Read the model definition and answer for the solid it produces. Units are mm, in the model's axes. Face numbers are marked on the shaded views. A direction names the side the tool comes from. Give positions to 0.01 mm unless a question says otherwise; leave off trailing zeros. Order: outer loops, then holes, each group sorted by start corner. A loop starts at its lowest first (then second) coordinate and runs counter-clockwise, first axis right, second up. Notation, with made-up numbers: (3, -11) - (16, -11) arc R18 cw to (16, 11) - close; hole circle Ø2 at (-3.75, 72). An arc over 180 degrees is marked (long way). Return JSON: item names as keys, results as strings.
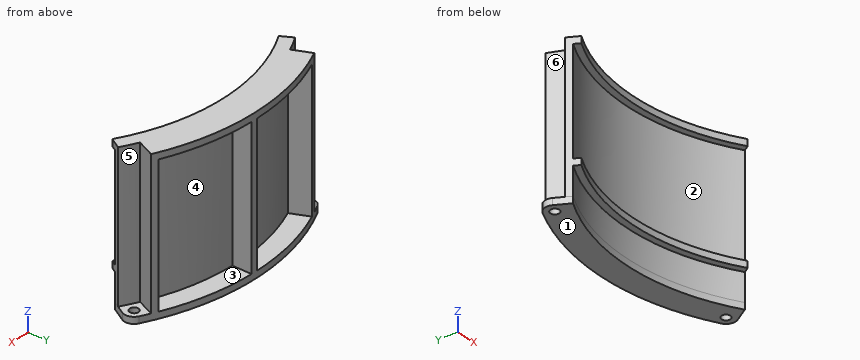
```python
from build123d import *

# Parameters (mm, degrees)
F1_DEPTH = 70.64375
F2_W     = 3.175
F2_H     = 50.8
F2_H_2   = 13.49375
F5_DEPTH = 70.64375
F6_R     = 2.15265
F7_DEPTH = 3.175
F9_DEPTH = 3.175


with BuildPart() as f1:
    # F0 (on Top) → F1 (new body)
    with BuildSketch(Plane.XY):
        with BuildLine():
            ThreePointArc((-49.2125, 85.2385503675), (0, 98.425), (49.2125, 85.2385503675))
            Line((49.2125, 85.2385503675), (57.15, 98.9867036526))
            ThreePointArc((57.15, 98.9867036526), (0, 114.3), (-57.15, 98.9867036526))
            Line((-57.15, 98.9867036526), (-49.2125, 85.2385503675))
        make_face()
    extrude(amount=F1_DEPTH)

    # F2 (on face) → F3 (revolve, cut)
    with BuildSketch(Plane(origin=(0, 0, 0), x_dir=(0.5, -0.8660254038, 0), z_dir=(-0.8660254038, -0.5, 0))):
        with Locations((-100.0125, 42.06875)):
            Rectangle(F2_W, F2_H)
        with Locations((-100.0125, 6.746875)):
            Rectangle(F2_W, F2_H_2)
    revolve(axis=Axis((0, 0, 0), (0, 0, -1)), mode=Mode.SUBTRACT)

    # F4 (on face) → F5 (cut, through all)
    with BuildSketch(Plane.XY.offset(70.64375)):
        with BuildLine():
            ThreePointArc((-48.2700740152, 103.6073836875), (-52.7606451092, 101.3943012583), (-57.15, 98.9867036526))
            Line((-57.15, 98.9867036526), (-52.3875, 90.7378116815))
            ThreePointArc((-52.3875, 90.7378116815), (-48.4225984878, 92.9142216277), (-44.3674611423, 94.9174853059))
            Line((-44.3674611423, 94.9174853059), (-48.2700740152, 103.6073836875))
        make_face()
        with BuildLine():
            Line((-45.3737460178, 104.9081177617), (-41.4711331449, 96.2182193801))
            ThreePointArc((-41.4711331449, 96.2182193801), (-21.9491383614, 102.4501632512), (-1.5875, 104.7629727945))
            Line((-1.5875, 104.7629727945), (-1.5875, 114.2889751627))
            ThreePointArc((-1.5875, 114.2889751627), (-23.944514576, 111.7638144558), (-45.3737460178, 104.9081177617))
        make_face()
        with BuildLine():
            Line((1.5875, 114.2889751627), (1.5875, 104.7629727945))
            ThreePointArc((1.5875, 104.7629727945), (21.9491383614, 102.4501632512), (41.4711331449, 96.2182193801))
            Line((41.4711331449, 96.2182193801), (45.3737460178, 104.9081177617))
            ThreePointArc((45.3737460178, 104.9081177617), (23.944514576, 111.7638144558), (1.5875, 114.2889751627))
        make_face()
        with BuildLine():
            ThreePointArc((44.3674611423, 94.9174853059), (48.4225984878, 92.9142216277), (52.3875, 90.7378116815))
            Line((52.3875, 90.7378116815), (57.15, 98.9867036526))
            ThreePointArc((57.15, 98.9867036526), (52.7606451092, 101.3943012583), (48.2700740152, 103.6073836875))
            Line((48.2700740152, 103.6073836875), (44.3674611423, 94.9174853059))
        make_face()
    extrude(amount=-F5_DEPTH, mode=Mode.SUBTRACT)

    # F6 (on face) → F7 (join)
    with BuildSketch(Plane(origin=(0, 0, 0), x_dir=(1, 0, 0), z_dir=(0, 0, -1))):
        with BuildLine():
            ThreePointArc((50.8, -87.9881810245), (0, -101.6), (-50.8, -87.9881810245))
            Line((-50.8, -87.9881810245), (-54.7169592083, -94.7725533844))
            ThreePointArc((-54.7169592083, -94.7725533844), (-55.1648447708, -98.4861661221), (-52.7921877107, -101.3778817924))
            ThreePointArc((-52.7921877107, -101.3778817924), (0, -114.3), (52.7921877107, -101.3778817924))
            ThreePointArc((52.7921877107, -101.3778817924), (55.1648447708, -98.4861661221), (54.7169592083, -94.7725533844))
            Line((54.7169592083, -94.7725533844), (50.8, -87.9881810245))
        make_face()
        with Locations((-50.5925132228, -97.1538033844)):
            Circle(F6_R, mode=Mode.SUBTRACT)
        with Locations((50.5925132228, -97.1538033844)):
            Circle(F6_R, mode=Mode.SUBTRACT)
    extrude(amount=F7_DEPTH)

    # F8 (on face) → F9 (join)
    with BuildSketch(Plane.XY.offset(70.64375)):
        with BuildLine():
            Line((44.3674611423, 94.9174853059), (48.2700740152, 103.6073836875))
            ThreePointArc((48.2700740152, 103.6073836875), (0, 114.3), (-48.2700740152, 103.6073836875))
            Line((-48.2700740152, 103.6073836875), (-44.3674611423, 94.9174853059))
            ThreePointArc((-44.3674611423, 94.9174853059), (0, 104.775), (44.3674611423, 94.9174853059))
        make_face()
    extrude(amount=-F9_DEPTH)


solid = f1.part
```
Q1. For the marked faces 1, 2 and 3, determine the directions among +Z, -Z, +X, -X, +Y, -Y from which every point of the face is accessible in a straight line to the end or side of a thin tool.
Values:
{"face 1": "-Z, +X, -X, +Y, -Y", "face 2": "-Y", "face 3": "+Y"}
Q2. Consider L1, parallel to Z at x = 26, y = 97.75; L2, parallel to Z at x = 24, y = 105 (3 decimals); L3, parallel to Y at x = -45, z = 4. Determine where each line is inside the solid, lowest interval first.
Values:
{"L1": "z = 13.49 to 16.67, 67.47 to 70.64", "L2": "z = -3.175 to 0, 67.469 to 70.644", "L3": "y = 91.09 to 94.62, 96.33 to 104.08"}
Q3. A cutting plane is placed at C-C (y = 107.25). Write down the section's boundary in (x, z) (1 decimal).
Values:
{"outline": "(-39.5, -3.2) - (39.5, -3.2) - (39.5, 0) - (1.6, 0) - (1.6, 67.5) - (39.5, 67.5) - (39.5, 70.6) - (-39.5, 70.6) - (-39.5, 67.5) - (-1.6, 67.5) - (-1.6, 0) - (-39.5, 0) - close"}
Q4. Determine the mould class of the marked faces 4, 5 and 6 for opening direction X: released by +X, released by -X, zero draft, split by the parting line, or undercut.
Values:
{"face 4": "undercut", "face 5": "released by +X", "face 6": "released by -X"}
Q5. A cutting plane is placed at B-B (x = -39.5). Write down the section's boundary in (y, z) (3 decimals).
Values:
{"outline": "(90.151, 13.494) - (93.607, 13.494) - (93.607, -3.175) - (107.258, -3.175) - (107.258, 0) - (97.044, 0) - (97.044, 67.469) - (107.258, 67.469) - (107.258, 70.644) - (90.151, 70.644) - (90.151, 67.469) - (93.607, 67.469) - (93.607, 16.669) - (90.151, 16.669) - close"}
Q6. Given pin 1 (4 mm diameter, centred on y = 100.5, z = 60, fed in from -X); pin 2 (7 mm diameter, centred on x = -50.59, y = 97.15, fed in from +Z); pin 3 (4 mm diameter, centred on y = 105.5, z = 61, fed in from +X), each flat-ended and moving along its own axis, determine where each tip first touches the part or whether it passes through.
Values:
{"pin 1": "stops at x = -47.77", "pin 2": "stops at z = 0", "pin 3": "stops at x = 48.27"}
Q7. A cutting plane is placed at D-D (x = -9.5). Write down the section's boundary in (y, z) (3 decimals).
Values:
{"outline": "(97.965, 13.494) - (101.155, 13.494) - (101.155, -3.175) - (113.905, -3.175) - (113.905, 0) - (104.343, 0) - (104.343, 67.469) - (113.905, 67.469) - (113.905, 70.644) - (97.965, 70.644) - (97.965, 67.469) - (101.155, 67.469) - (101.155, 16.669) - (97.965, 16.669) - close"}
